Check sheet for the drawn part. Datum: minimum x, y, z corner. Units: mm. A direction names the side the tool comes from. Round coordinates to 2 decimals unless told otherwise and drop trailing zeros. Write each loop counter-clockwise with the first axis right and the second up, starting at its lowest first coordinate (ties: lowest second). Pieces come first, ordered by that corner, then holes. Notation, with made-up numbers: M -33.5,-37 L -27.5,-37 A15 cw -27.5,-24 Z; hole C 61,41 d11. An arc over 180 degrees is marked long. One line per item, written item: value. Start each with the question number.
Item 1: Section check C-C, the plane x = 37.16. Record the cut outline in (y, z).
Item 2: Section check A-A, the plane z = 4.25. Record the cut outline in (x, y), then the cut area to 3 significant figures.
Item 3: Thickness scan on probe 1 along Y at (x, z) = (6.84, 6.25); probe 2 along Y at (x, z) = (37.16, 9); probe 3 along X at (y, z) = (8, 5.5). Record the ranges inside material, lowest first. Write a range as from..to.
Item 4: Section check D-D, the plane x = 4. Record the cut outline in (y, z).
Item 5: Section check B-B, the plane y = 6.75. Record the cut outline in (x, z).
Item 6: Gauge pin test, flat ends, axial feed: pin 1 (8 mm diameter, centred on x = 39, y = 37, fed in from +Z); pin 2 (3.5 mm diameter, centred on x = 6.84, y = 37.25, fed in from -Z); pin 3 (2.5 mm diameter, centred on x = 21, z = 13.5, fed in from +Y); pin 4 (2.5 mm diameter, centred on y = 19, z = 12, fed in from -X). Record the tip position at first contact, or that the pin passes through.
Item 7: Tool access check on the marked faces 1, 2, 3, 4 and 5. Record the directions out of +Z, -Z, +X, -X, +Y, -Y that give a thin tool (end or side, any length) a straight path to the whole face; none if there is none.
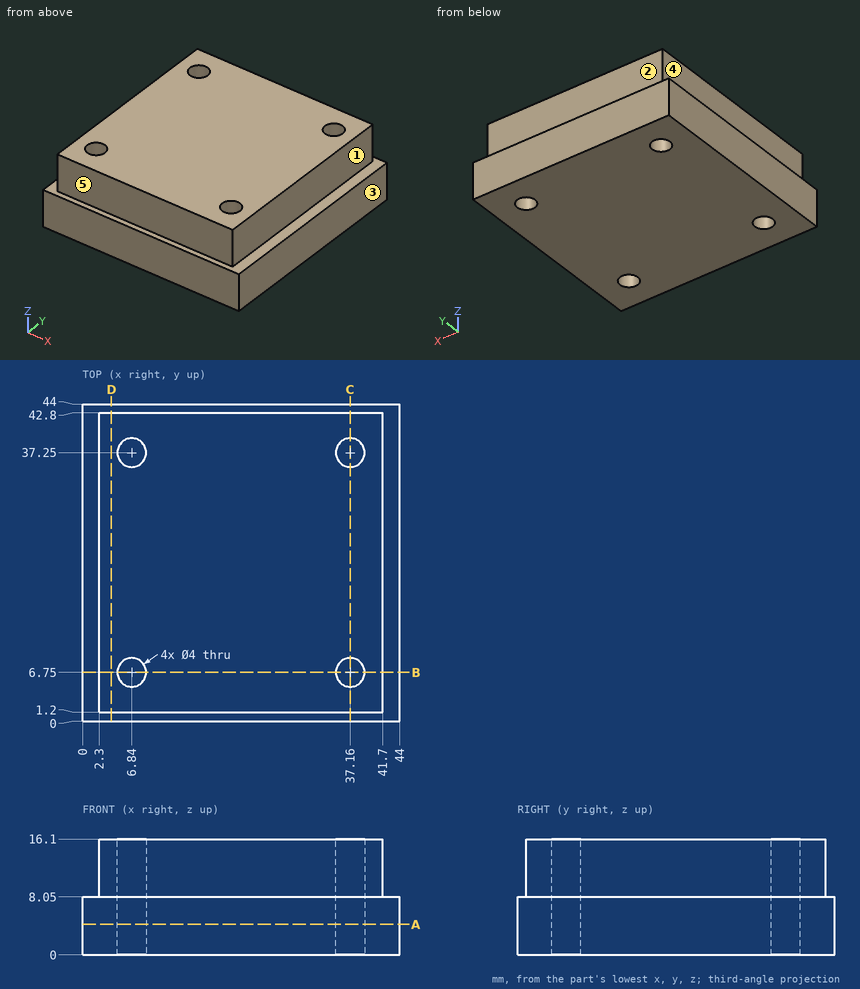
Response values:
1. outline: M 0,0 L 4.75,0 L 4.75,16.1 L 1.2,16.1 L 1.2,8.05 L 0,8.05 Z; M 8.75,0 L 35.25,0 L 35.25,16.1 L 8.75,16.1 Z; M 39.25,0 L 44,0 L 44,8.05 L 42.8,8.05 L 42.8,16.1 L 39.25,16.1 Z
2. outline: M 0,0 L 44,0 L 44,44 L 0,44 Z; hole C 6.84,6.75 d4; hole C 6.84,37.25 d4; hole C 37.16,6.75 d4; hole C 37.16,37.25 d4
2. area: 1,890 mm2
3. probe 1: y = 0..4.75, 8.75..35.25, 39.25..44
3. probe 2: y = 1.2..4.75, 8.75..35.25, 39.25..42.8
3. probe 3: x = 0..5.28, 8.4..35.6, 38.72..44
4. outline: M 0,0 L 44,0 L 44,8.05 L 42.8,8.05 L 42.8,16.1 L 1.2,16.1 L 1.2,8.05 L 0,8.05 Z
5. outline: M 0,0 L 4.84,0 L 4.84,16.1 L 2.3,16.1 L 2.3,8.05 L 0,8.05 Z; M 8.84,0 L 35.16,0 L 35.16,16.1 L 8.84,16.1 Z; M 39.16,0 L 44,0 L 44,8.05 L 41.7,8.05 L 41.7,16.1 L 39.16,16.1 Z
6. pin 1: stops at z = 16.1
6. pin 2: passes through
6. pin 3: stops at y = 42.8
6. pin 4: stops at x = 2.3
7. face 1: +Z, +X, +Y, -Y
7. face 2: +Z, +X, -X, +Y
7. face 3: +Z, -Z, +X, +Y, -Y
7. face 4: +Z, -X, +Y, -Y
7. face 5: +Z, +X, -X, -Y
